Geometry: see drawing. Coordinates: mm, zero at the bounding-box minimum. A direction names the side the tool comes from. Coordinates: 2 decimals unless noted, no trailing zeros. Order: outer loops, then holes, each group sorted by start corner. A loop starts at its lowest first (then second) coordinate and runs counter-clockwise, first axis right, second up. Notation, with made-up numbers: (21, -8) -> (29, -8) arc R17 ccw to (29, 9) -> close; hole circle Ø10 at (3.5, 78.5). An arc over 180 degrees is marked (long way). Use one line per item in the form item = value.
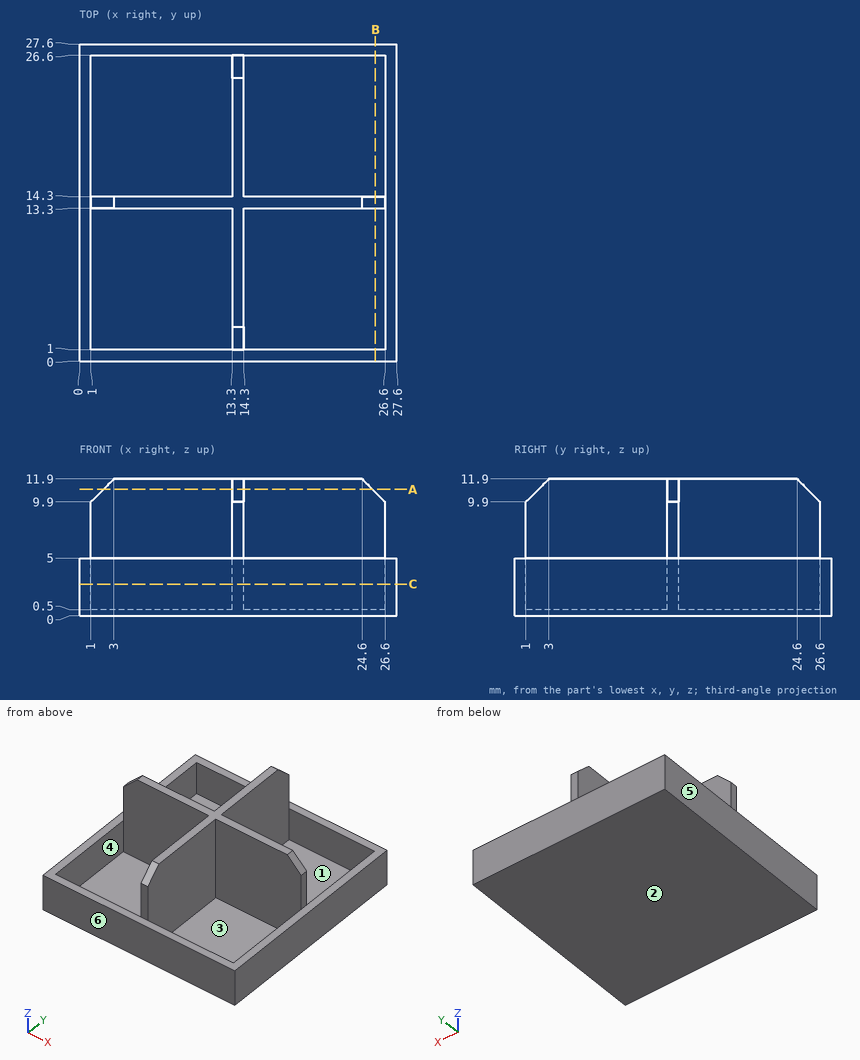
1) Section A-A, the plane z = 11. Output: boundary loops of the cut face in (x, y), and give its area (3 significant figures).
Results found:
outline = (2.1, 13.3) -> (13.3, 13.3) -> (13.3, 2.1) -> (14.3, 2.1) -> (14.3, 13.3) -> (25.5, 13.3) -> (25.5, 14.3) -> (14.3, 14.3) -> (14.3, 25.5) -> (13.3, 25.5) -> (13.3, 14.3) -> (2.1, 14.3) -> close
area = 45.8 mm2
2) Material intervals for probe 1 along X at (y, z) = (5.5, 3); probe 2 along Y at (x, z) = (14.75, 8.75), sorted ascending. Write a range as from..to.
Results found:
probe_1 = 0..1, 13.3..14.3, 26.6..27.6
probe_2 = 13.3..14.3
3) Section B-B, the plane x = 25.75. Output: boundary loops of the cut face in (y, z).
Results found:
outline = (0, 0) -> (27.6, 0) -> (27.6, 5) -> (26.6, 5) -> (26.6, 0.5) -> (14.3, 0.5) -> (14.3, 10.75) -> (13.3, 10.75) -> (13.3, 0.5) -> (1, 0.5) -> (1, 5) -> (0, 5) -> close
4) Pull-direction query (X, two-part tool) for the marked faces 3, 4, 5 and 6; classes: released by +X, released by -X, zero draft, split by the parting line, or undercut.
Results found:
face_3 = undercut
face_4 = undercut
face_5 = released by -X
face_6 = zero draft
5) Contact query for flat-ended pins moving along their axis: P1, Ø0.5, axis at y = 13.5, z = 8.5, coming from the +X side; P2, Ø13.5, axis at x = 6, y = 22, coming from the +Z side; P3, Ø1.1, axis at y = 13.5, z = 6.5, coming from the -X side. Output: stop coordinate, or through.
Results found:
P1 = 26.6
P2 = 5
P3 = 1
6) Section C-C, the plane z = 2.75. Output: boundary loops of the cut face in (x, y).
Results found:
outline = (0, 0) -> (27.6, 0) -> (27.6, 27.6) -> (0, 27.6) -> close; hole (1, 1) -> (13.3, 1) -> (13.3, 13.3) -> (1, 13.3) -> close; hole (1, 14.3) -> (13.3, 14.3) -> (13.3, 26.6) -> (1, 26.6) -> close; hole (14.3, 1) -> (26.6, 1) -> (26.6, 13.3) -> (14.3, 13.3) -> close; hole (14.3, 14.3) -> (26.6, 14.3) -> (26.6, 26.6) -> (14.3, 26.6) -> close
7) Access query for the marked faces 1 and 2. Directions: +Z, -Z, +X, -X, +Y, -Y. A direction counts if a zero-diameter tool reaches every point of the face in a straight line with its end or side. Return the directions, or none.
Results found:
face_1 = +Z
face_2 = -Z, +X, -X, +Y, -Y
